Autodesk Inventor part; units mm, degrees
ref_plane "YZ Plane" through (0, 0, 0) normal (1, 0, 0) x (0, 1, 0)
ref_plane "XZ Plane" through (0, 0, 0) normal (0, 1, 0) x (-1, 0, 0)
ref_plane "XY Plane" through (0, 0, 0) normal (0, 0, 1) x (1, 0, 0)
sketch "スケッチ1" plane through (0, 0, 0) normal (0, 0, 1) x (1, 0, 0)
  line L0 (-37.5, 9.6) -> (-37.5, 16.25)
  line L1 (-37.5, 16.25) -> (-20, 16.25)
  line L2 (20, 16.25) -> (37.5, 16.25)
  line L3 (37.5, 16.25) -> (37.5, 9.6)
  line L4 (0, 0) -> (0, 16.25) construction
  line L5 (0, 0) -> (39.5, 0) construction
  line L6 (37.5, 7.5) -> (39.5, 7.5)
  line L7 (39.5, 7.5) -> (39.5, -7.5)
  line L8 (39.5, -7.5) -> (37.5, -7.5)
  line L9 (-20, -16.25) -> (20, -16.25) construction
  line L10 (20, -16.25) -> (20, 16.25) construction
  line L11 (20, 16.25) -> (-20, 16.25) construction
  line L12 (-20, 16.25) -> (-20, -16.25) construction
  line L13 (-20, -16.25) -> (20, 16.25) construction
  line L14 (20, -16.25) -> (-20, 16.25) construction
  line L15 (-37.5, -16.25) -> (37.5, -16.25) construction
  line L16 (37.5, -16.25) -> (37.5, 16.25) construction
  line L17 (37.5, 16.25) -> (-37.5, 16.25) construction
  line L18 (-37.5, 16.25) -> (-37.5, -16.25) construction
  line L19 (-37.5, -16.25) -> (37.5, 16.25) construction
  line L20 (37.5, -16.25) -> (-37.5, 16.25) construction
  arc A0 (37.5, 9.6) -> (37.5, 7.5) centre (37.5, 8.55) ccw
  arc A1 (37.5, -7.5) -> (37.5, -9.6) centre (37.5, -8.55) ccw
  line L21 (37.5, -9.6) -> (37.5, -16.25)
  line L22 (37.5, -16.25) -> (20, -16.25)
  line L23 (20, -16.25) -> (12.1, -16.25)
  line L24 (-20, 16.25) -> (-12.1, 16.25)
  line L25 (-10, 16.25) -> (-10, 18.25)
  line L26 (-10, 18.25) -> (10, 18.25)
  line L27 (10, 18.25) -> (10, 16.25)
  line L28 (20, 16.25) -> (12.1, 16.25)
  arc A2 (-12.1, 16.25) -> (-10, 16.25) centre (-11.05, 16.25) ccw
  arc A3 (10, 16.25) -> (12.1, 16.25) centre (11.05, 16.25) ccw
  line L29 (-37.5, 7.5) -> (-39.5, 7.5)
  line L30 (-39.5, 7.5) -> (-39.5, -7.5)
  line L31 (-39.5, -7.5) -> (-37.5, -7.5)
  arc A4 (-37.5, 7.5) -> (-37.5, 9.6) centre (-37.5, 8.55) ccw
  arc A5 (-37.5, -9.6) -> (-37.5, -7.5) centre (-37.5, -8.55) ccw
  line L32 (-37.5, -9.6) -> (-37.5, -16.25)
  line L33 (-37.5, -16.25) -> (-20, -16.25)
  line L34 (-20, -16.25) -> (-12.1, -16.25)
  line L35 (-10, -16.25) -> (-10, -18.25)
  line L36 (-10, -18.25) -> (10, -18.25)
  line L37 (10, -18.25) -> (10, -16.25)
  arc A6 (-10, -16.25) -> (-12.1, -16.25) centre (-11.05, -16.25) ccw
  arc A7 (12.1, -16.25) -> (10, -16.25) centre (11.05, -16.25) ccw
  line L38 (-16.55, 19.1799) -> (-13.45, 19.1799) construction
  line L39 (-13.45, 19.1799) -> (-13.45, 12.4242) construction
  line L40 (-13.45, 12.4242) -> (-16.55, 12.4242) construction
  line L41 (-16.55, 12.4242) -> (-16.55, 19.1799) construction
  line L42 (-15, 19.1799) -> (-15, 12.4242) construction
  point P0 (0, 18.25)
  point P1 (0, 0)
  dimension "d0" = 1.05
  dimension "d1" = 32.5
  dimension "d2" = 75
  dimension "d3" = 40
  dimension "d23" = 2
  dimension "d30" = 2
  dimension "d34" = 8.75
  dimension "d53" = 20
  dimension "d54" = 3.1
  dimension "d55" = 5
  dimension "d85" = 32.5
extrude "押し出し1" add sketch "スケッチ1" along normal blind 5
sketch "スケッチ2" plane through (0, 0, 0) normal (0, 0, -1) x (-1, 0, 0)
  line L0 (37.5, 9.6) -> (37.5, 16.25)
  line L1 (-37.5, 16.25) -> (-37.5, 9.6)
  line L2 (-45.6427, 17.3125) -> (-37.5, 17.3125)
  line L3 (-37.5, 17.3125) -> (-37.5, -16.751)
  line L4 (-37.5, -16.751) -> (-45.6427, -16.751)
  line L5 (-45.6427, -16.751) -> (-45.6427, 17.3125)
  line L6 (37.5, 21.1805) -> (43.358, 21.1805)
  line L7 (43.358, 21.1805) -> (43.358, -13.6193)
  line L8 (43.358, -13.6193) -> (37.5, -13.6193)
  line L9 (37.5, -13.6193) -> (37.5, 21.1805)
  line L10 (-20, -16.25) -> (-12.1, -16.25)
  line L11 (-17.1371, 25.1848) -> (11.8342, 25.1848)
  line L12 (11.8342, 25.1848) -> (11.8342, 16.25)
  line L13 (11.8342, 16.25) -> (-17.1371, 16.25)
  line L14 (-17.1371, 16.25) -> (-17.1371, 25.1848)
  line L15 (-13.151, -21.5857) -> (17.7795, -21.5857)
  line L16 (17.7795, -21.5857) -> (17.7795, -16.25)
  line L17 (17.7795, -16.25) -> (-13.151, -16.25)
  line L18 (-13.151, -16.25) -> (-13.151, -21.5857)
  line L19 (-12.1, 16.25) -> (-37.5, 16.25)
  line L20 (-37.5, -16.25) -> (-12.1, -16.25)
  point P0 (0, 0)
extrude "押し出し2" cut sketch "スケッチ2" against normal blind 2.5
sketch "スケッチ3" plane through (12.1, 16.25, 0) normal (0, 1, 0) x (1, 0, 0)
  line L0 (-2.1, 0) -> (-2.1, -5)
  line L1 (-2.1, -5) -> (-22.1, -5) construction
  line L2 (-12.1, -5) -> (-12.1, 7.4607) construction
  line L3 (25.4, 0) -> (25.4, -5)
  point P0 (-12.1, 0)
  point P1 (2.9, -2.5)
  point P2 (-27.1, -2.5)
  point P3 (25.4, -2.5)
  dimension "d60" = 5
hole "穴1" at (15, 16.25, 2.5) at (-15, 16.25, 2.5) direction (0, -1, 0) diameter 2.459 depth 2.5
mirror "ミラー1" about plane through (0, 0, 0) normal (0, 1, 0) of "穴1"
sketch "スケッチ4" plane through (37.5, -16.25, 5) normal (1, 0, 0) x (0, 0, -1)
  line L0 (5, 16.25) -> (0, 16.25) construction
  line L1 (0, 23.75) -> (0, 8.75) construction
  line L2 (5, 6.65) -> (0, 6.65)
  line L3 (5, 0) -> (0, 0)
  point P0 (2.5, 3)
  point P1 (2.5, 29.5)
  point P2 (2.5, 6.65)
  dimension "d86" = 3
  dimension "d87" = 26.5
hole "穴2" at (37.5, -13.25, 2.5) at (37.5, 13.25, 2.5) direction (-1, 0, 0) diameter 2.459 depth 2.5
mirror "ミラー2" about plane through (0, 0, 0) normal (1, 0, 0) of "穴2"
sketch "スケッチ5" plane through (0, 0, 0) normal (0, 0, -1) x (-1, 0, 0)
  line L0 (10, 16.25) -> (-10, 16.25)
  line L1 (-37.5, 7.5) -> (-37.5, 9.6)
  line L2 (-32.5, -11.25) -> (32.5, -11.25) construction
  line L3 (32.5, -11.25) -> (32.5, 11.25) construction
  line L4 (32.5, 11.25) -> (-32.5, 11.25) construction
  line L5 (-32.5, 11.25) -> (-32.5, -11.25) construction
  line L6 (-32.5, -11.25) -> (32.5, 11.25) construction
  line L7 (32.5, -11.25) -> (-32.5, 11.25) construction
  line L8 (-32.5, 9.1336) -> (-32.5, -9.1336)
  line L9 (-32.5, -9.1336) -> (-6.1141, 0)
  line L10 (-6.1141, 0) -> (-32.5, 9.1336)
  line L11 (-26.3859, 11.25) -> (26.3859, 11.25)
  line L12 (26.3859, 11.25) -> (0, 2.1164)
  line L13 (0, 2.1164) -> (-26.3859, 11.25)
  line L14 (-26.3859, -11.25) -> (26.3859, -11.25)
  line L15 (26.3859, -11.25) -> (0, -2.1164)
  line L16 (0, -2.1164) -> (-26.3859, -11.25)
  line L17 (32.5, 9.1336) -> (32.5, -9.1336)
  line L18 (32.5, -9.1336) -> (6.1141, 0)
  line L19 (6.1141, 0) -> (32.5, 9.1336)
  point P0 (-12.1, 16.25)
  point P1 (-20, 16.25)
  point P2 (-37.5, 16.25)
  point P3 (0, 0)
  dimension "d76" = 5
  dimension "d77" = 5
  dimension "d78" = 4
  dimension "d79" = 4
  dimension "d80" = 4
  dimension "d81" = 4
extrude "押し出し3" cut sketch "スケッチ5" against normal blind 10
fillet "フィレット1" radius 1.05 12 edges at (32.5, 9.1336, 2.5) (32.5, -9.1336, 2.5) (26.3859, 11.25, 2.5) (6.1141, 0, 2.5) (0, -2.1164, 2.5) (0, 2.1164, 2.5) (-32.5, -9.1336, 2.5) (26.3859, -11.25, 2.5) (-32.5, 9.1336, 2.5) (-26.3859, 11.25, 2.5) (-26.3859, -11.25, 2.5) (-6.1141, 0, 2.5)
equation "\"d85\" = d1"
equation "\"d77\" = d76"
equation "\"d79\" = d78"
equation "\"d80\" = d79"
equation "\"d81\" = d78"
equation "\"d48\" = 26.5"
equation "\"d52\" = 5"
properties part number "Trunk_horizontal_frame_04" material "アセタール樹脂、黒"
The model under review builds one solid part; all positions refer to its coordinate system, in mm. A direction names the side the tool comes from. Give positions to 0.01 mm unless a question says otherwise; leave off trailing zeros. Order: outer loops, then holes, each group sorted by start corner. A loop starts at its lowest first (then second) coordinate and runs counter-clockwise, first axis right, second up. Notation, with made-up numbers: M 46.5,-31.5 L 99.5,-31.5 A10 cw 99.5,-13.5 Z; hole C 32.25,-34.75 d11. An arc over 180 degrees is marked long. One line per question, with ' | ' between items. Start each with the question number.
1) Consider section A-A, the plane x = 18. Give the boundary of the cut face in (y, z), then the cut area to 3 significant figures.
2) Consider section D-D, the plane x = 34. Give the boundary of the cut face in (y, z).
3) Consider section B-B, the plane x = -3.5. Give the boundary of the cut face in (y, z).
4) Clearance check with flat-ended pins moving along their axes: P1, Ø2, axis at x = 15, z = 2.5, coming from the -Y side; P2, Ø0.6, axis at x = -38.5, z = 4, coming from the -Y side; P3, Ø1.5, axis at x = 8, z = 1.5, coming from the +Y side. State where each tip first meets the part, or that it passes through.
5) Mouldability with a two-part tool opening along X and no side actions: class faces 4 (the face through (0, -18.25, 4)), 5 (the face through (8.274, 0.018, 2.535)), 6 (the face through (36.45, 8.53, 2.46)) as pulls with the +X half, pulls with the -X half, needs draft (parallel to the pull), parting line crosses it, or undercut.
6) For faces 1 (the face through (-38, 7.5, 4)), 2 (the face through (37.5, 0, 1)), 3 (the face through (10, -17, 4)), list the 3-axis set-ups (+Z, -Z, +X, -X, +Y, -Y) from which the entire face can be reached by the end or side of a thin tool; tool diameter is ignored.
7) Wall thickness on L1, parallel to Z at x = -36.5, y = 13.25; L2, parallel to X at y = 14, z = 1.85; L3, parallel to Y at x = -19, z = 4.15: over which ranges is each line inside the solid? List them lowest first. Write a range as from..to.
8) Consider section C-C, the plane x = -22.5. Give the boundary of the cut face in (y, z).
Found:
1) outline: M -16.25,0 L -11.25,0 L -11.25,5 L -16.25,5 Z; M -8.35,0 L -4.11,0 L -4.11,5 L -8.35,5 Z; M 4.11,0 L 8.35,0 L 8.35,5 L 4.11,5 Z; M 11.25,0 L 16.25,0 L 16.25,5 L 11.25,5 Z | area: 92.3 mm²
2) outline: M -16.25,0 L 16.25,0 L 16.25,5 L -16.25,5 Z
3) outline: M -18.25,2.5 L -16.25,2.5 L -16.25,0 L -11.25,0 L -11.25,5 L -18.25,5 Z; M -3.33,0 L 3.33,0 L 3.33,5 L -3.33,5 Z; M 11.25,0 L 16.25,0 L 16.25,2.5 L 18.25,2.5 L 18.25,5 L 11.25,5 Z
4) P1: stops at y = -13.75 | P2: stops at y = -7.5 | P3: stops at y = 16.25
5) face 4: needs draft | face 5: undercut | face 6: pulls with the +X half
6) face 1: +Z, -Z, -X, +Y | face 2: -Z, +X, +Y, -Y | face 3: +Z, -Z, +X, -Y
7) L1: z = 0..1.27, 3.73..5 | L2: x = -35..-16.04, -13.96..13.96, 16.04..35 | L3: y = -16.25..-11.25, -8.69..-4.46, 4.46..8.69, 11.25..16.25
8) outline: M -16.25,0 L -5.67,0 L -5.67,5 L -16.25,5 Z; M 5.67,0 L 16.25,0 L 16.25,5 L 5.67,5 Z
